CAD build for the part. Positions are in the model's coordinates, mm. A direction names the side the tool comes from. Round coordinates to 2 decimals unless told otherwise and drop trailing zeros. Loops run counter-clockwise (first coordinate to the right, second up) from the corner with the lowest first, then second, coordinate; pieces in that order, holes last. Notation, with made-up numbers: M 89.5,12.25 L 109.5,12.25 A33 cw 109.5,51.25 Z; hole C -28.5,81.25 d9. An arc over 180 degrees is marked long. Use one line per item in the form item = value.
from build123d import *

# Parameters (mm, degrees)
SKETCH1_W           = 533.4
SKETCH1_H           = 279.4
BOSS_EXTRUDE1_DEPTH = 6.35
SKETCH2_W           = 482.6
SKETCH2_H           = 6.35
CUT_EXTRUDE1_DEPTH  = 302.34078715
SKETCH3_W           = 19.05
SKETCH3_H           = 158.75
CUT_EXTRUDE2_DEPTH  = 302.34078715
SKETCH4_W           = 17.4498
SKETCH4_H           = 51.59375
CUT_EXTRUDE3_DEPTH  = 302.34078715
SKETCH5_W           = 54.76875
SKETCH5_H           = 28.575
CUT_EXTRUDE4_DEPTH  = 302.34078715
SKETCH6_W           = 154.4828
SKETCH6_H           = 4.6
CUT_EXTRUDE5_DEPTH  = 6.35


with BuildPart() as part:
    # Sketch1 → Boss-Extrude1 (new, symmetric)
    with BuildSketch(Plane(origin=(0, 0, 0), x_dir=(1, 0, 0), z_dir=(0, 1, 0))):
        Rectangle(SKETCH1_W, SKETCH1_H)
    extrude(amount=BOSS_EXTRUDE1_DEPTH, both=True)

    # Sketch2 → Cut-Extrude1 (cut, through all)
    with BuildSketch(Plane(origin=(0, 6.35, 0), x_dir=(1, 0, 0), z_dir=(0, 1, 0))):
        with Locations((0, 136.525)):
            Rectangle(SKETCH2_W, SKETCH2_H)
    extrude(amount=-CUT_EXTRUDE1_DEPTH, mode=Mode.SUBTRACT)

    # Sketch3 → Cut-Extrude2 (cut, through all)
    with BuildSketch(Plane(origin=(0, 6.35, 0), x_dir=(1, 0, 0), z_dir=(0, 1, 0))):
        with Locations((-101.6, 53.975)):
            Rectangle(SKETCH3_W, SKETCH3_H)
        with Locations((101.6, 53.975)):
            Rectangle(SKETCH3_W, SKETCH3_H)
    extrude(amount=-CUT_EXTRUDE2_DEPTH, mode=Mode.SUBTRACT)

    # Sketch4 → Cut-Extrude3 (cut, through all)
    with BuildSketch(Plane(origin=(0, 6.35, 0), x_dir=(1, 0, 0), z_dir=(0, 1, 0))):
        Polygon((165.1254, 73.025), (250.8504, 73.025), (250.8504, 34.925), (165.1254, 34.925), (165.1254, 28.178125), (155.6004, 28.178125), (155.6004, 79.771875), (165.1254, 79.771875), align=None)
        with Locations((-83.3501, 53.975)):
            Rectangle(SKETCH4_W, SKETCH4_H)
        with Locations((83.3501, 53.975)):
            Rectangle(SKETCH4_W, SKETCH4_H)
    extrude(amount=-CUT_EXTRUDE3_DEPTH, mode=Mode.SUBTRACT)

    # Sketch5 → Cut-Extrude4 (cut, through all)
    with BuildSketch(Plane(origin=(0, 6.35, 0), x_dir=(1, 0, 0), z_dir=(0, 1, 0))):
        with Locations((0, 119.0625)):
            Rectangle(SKETCH5_W, SKETCH5_H)
    extrude(amount=-CUT_EXTRUDE4_DEPTH, mode=Mode.SUBTRACT)

    # Sketch6 → Cut-Extrude5 (cut)
    with BuildSketch(Plane(origin=(0, 6.35, 0), x_dir=(1, 0, 0), z_dir=(0, 1, 0))):
        with Locations((-189.4586, -127.675)):
            Rectangle(SKETCH6_W, SKETCH6_H)
        with Locations((-189.4586, 8.85)):
            Rectangle(SKETCH6_W, SKETCH6_H)
        with Locations((-189.4586, 118.15)):
            Rectangle(SKETCH6_W, SKETCH6_H)
        with Locations((-189.4586, -8.85)):
            Rectangle(SKETCH6_W, SKETCH6_H)
    cut_extrude5 = extrude(amount=-CUT_EXTRUDE5_DEPTH, mode=Mode.SUBTRACT)

    # Mirror1: Cut-Extrude5 across plane
    add(cut_extrude5.mirror(Plane(origin=(0, 0, 0), x_dir=(0, 0, 1), z_dir=(1, 0, 0))), mode=Mode.SUBTRACT)


solid = part.part
1. Cut at D-D on x = -21.5. Write the cut outline in (y, z) (3 decimals).
Completed:
outline = M -6.35,-104.775 L 6.35,-104.775 L 6.35,139.7 L -6.35,139.7 Z
2. Tool access for faces 1 (the face through (266.7, 0, 2)), 2 (the face through (160, 0, -79.772)), 3 (the face through (-111.125, 0, -53)): list every direction of +Z, -Z, +X, -X, +Y, -Y with a clear straight run to the whole face (end or side of a thin tool).
Completed:
face_1 = +Z, -Z, +X, +Y, -Y
face_2 = +Y, -Y
face_3 = -Z, +Y, -Y
3. Pull direction Z, two halves, no side cores. Call faces 4 (the face through (-83, 0, -28.178)), 5 (the face through (250.85, 0, -54)), 6 (the face through (-4, 0, 139.7)), 7 (the face through (59, 0, -133.35)): +Z half, -Z half, draft (parallel to the pull), parting line (faces both ways), or undercut.
Completed:
face_4 = undercut
face_5 = undercut
face_6 = +Z half
face_7 = -Z half
4. Probe line 1 along X through (y, z) = (5.5, 5) (3 decimals); line 2 along Z through (x, y) = (183.5, 4.75) (3 decimals); line 3 along X through (y, z) = (-4.5, -52) (3 decimals). List the from-to ranges inside material, lowest first. Write a range as from..to.
Completed:
line_1 = -266.7..-111.125, -92.075..92.075, 111.125..266.7
line_2 = -133.35..-120.45, -115.85..-73.025, -34.925..-11.15, -6.55..6.55, 11.15..125.375, 129.975..139.7
line_3 = -266.7..-111.125, -74.625..74.625, 111.125..155.6, 250.85..266.7
5. Cut at C-C on x = 51.5. Write the cut outline in (y, z).
Completed:
outline = M -6.35,-133.35 L 6.35,-133.35 L 6.35,139.7 L -6.35,139.7 Z
6. Cut at A-A on z = -99. Write the cut outline in (x, y) (3 decimals).
Completed:
outline = M -266.7,-6.35 L -111.125,-6.35 L -111.125,6.35 L -266.7,6.35 Z; M -92.075,-6.35 L 92.075,-6.35 L 92.075,6.35 L -92.075,6.35 Z; M 111.125,-6.35 L 266.7,-6.35 L 266.7,6.35 L 111.125,6.35 Z
7. Cut at B-B on x = -201. Write the cut outline in (y, z) (3 decimals).
Completed:
outline = M -6.35,-133.35 L 6.35,-133.35 L 6.35,-120.45 L 0,-120.45 L 0,-115.85 L 6.35,-115.85 L 6.35,-11.15 L 0,-11.15 L 0,-6.55 L 6.35,-6.55 L 6.35,6.55 L 0,6.55 L 0,11.15 L 6.35,11.15 L 6.35,125.375 L 0,125.375 L 0,129.975 L 6.35,129.975 L 6.35,139.7 L -6.35,139.7 Z
8. Drop flat-ended pins along their axis: P1, Ø6.5, axis at x = -104, y = -2.5, coming from the -Z side; P2, Ø1.4, axis at y = 2.5, z = 127, coming from the +X side; P3, Ø5, axis at x = -203, z = -8, coming from the +Y side; P4, Ø1.4, axis at y = 3, z = -119, coming from the -X side. Give the stop position or say it passes through.
Completed:
P1 = 25.4
P2 = 112.22
P3 = 6.35
P4 = -112.22
